Source: three-view drawing plus pictorial views. Frame: mm from the lowest corner of the part. A direction names the side the tool comes from. Round coordinates to 2 decimals unless told otherwise and drop trailing zeros. Order: outer loops, then holes, each group sorted by start corner. A loop starts at its lowest first (then second) coordinate and runs counter-clockwise, first axis right, second up. Notation, with made-up numbers: (17.25, 48) -> (38.25, 48) arc R19 ccw to (38.25, 55) -> close; hole circle Ø3 at (86.5, 15). An arc over 180 degrees is marked (long way). Answer as CSV lines item,"result". Start each with the question number.
1) Line query: L1, parallel to Y at x = 9.5, z = 22.8; L2, parallel to Y at x = 9.5, z = 9.75; L3, parallel to Z at x = 4.75, y = 17. Output: solid intervals per line, ascending.
2) Section query D-D, the plane z = 2.5. Output: boundary loops of the cut face in (x, y), and give its area (3 significant figures).
3) Access query for the marked faces 4 and 5. Directions: +Z, -Z, +X, -X, +Y, -Y. A direction counts if a zero-diameter tool reaches every point of the face in a straight line with its end or side. Return the directions, or none.
4) First-contact query: P1, Ø5.5, axis at x = 9.5, y = 9.5, coming from the -Z side; P2, Ø1, axis at y = 8, z = 13.5, coming from the +X side; P3, Ø3.5, axis at x = 11, y = 8, coming from the -Z side. Flat tips, straight axial feed; report the tip coordinate or a pass-through.
5) Section query B-B, the plane z = 21.25. Output: boundary loops of the cut face in (x, y).
6) Mould query, pull axis Y, two halves, no side actions, for the marked faces 1, 2 and 3. Classes: +Y half, -Y half, draft (parallel to the pull), parting line (faces both ways), or undercut.
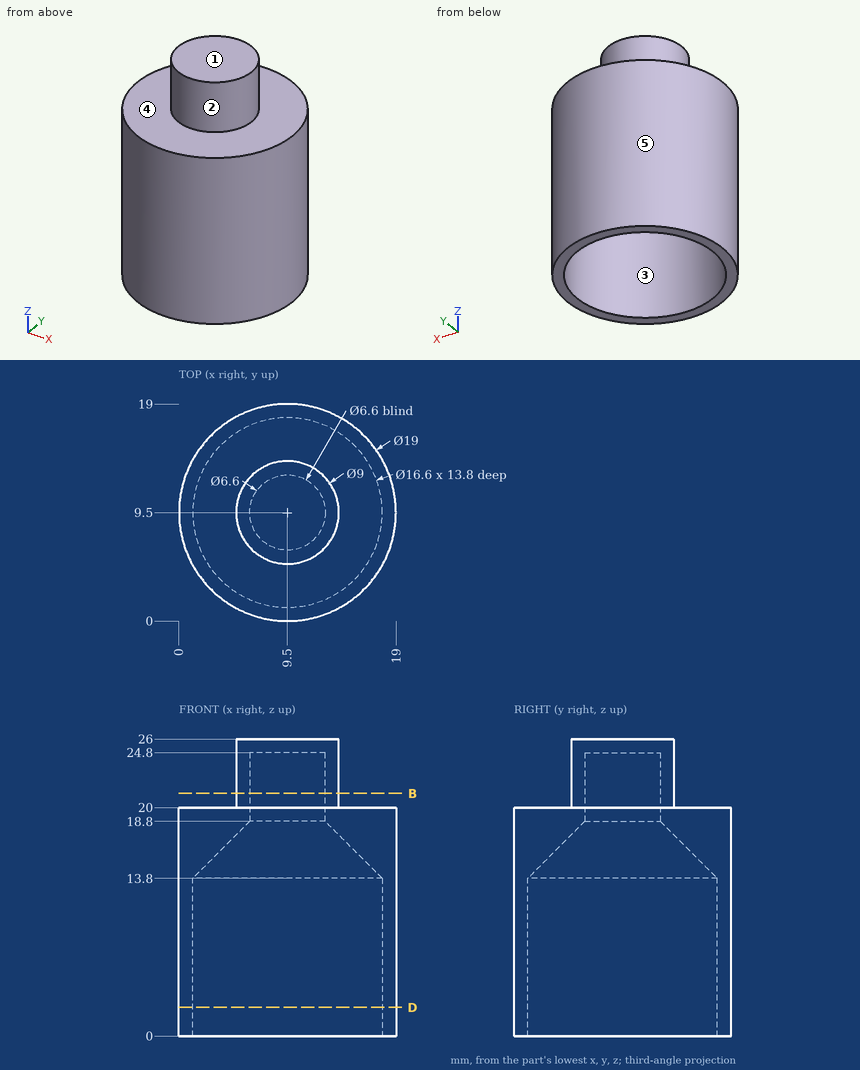
Findings:
1,L1,"y = 5 to 6.2, 12.8 to 14"
1,L2,"y = 0 to 1.2, 17.8 to 19"
1,L3,"z = 0 to 20"
2,outline,"circle Ø19 at (9.5, 9.5); hole circle Ø16.6 at (9.5, 9.5)"
2,area,"67.1 mm^2"
3,face 4,"+Z"
3,face 5,"+Z, -Z"
4,P1,"stops at z = 24.8"
4,P2,"stops at x = 18.95"
4,P3,"stops at z = 18.23"
5,outline,"circle Ø9 at (9.5, 9.5); hole circle Ø6.6 at (9.5, 9.5)"
6,face 1,"draft"
6,face 2,"parting line"
6,face 3,"undercut"
